For this review, use the dimensioned drawing (mm, ordinates from the lowest corner) and the shaded views. A direction names the side the tool comes from. Coordinates: 2 decimals unless noted, no trailing zeros. Write each loop counter-clockwise with the first axis right and the second up, starting at its lowest first coordinate (ties: lowest second). Pieces come first, ordered by that corner, then holes. Notation, with made-up numbers: (-34.75, 38.5) - (-30.75, 38.5) arc R22 ccw to (-30.75, 44.5) - close; hole circle Ø6 at (-13.5, 65). An arc over 180 degrees is marked (long way). One line per item, written item: value.
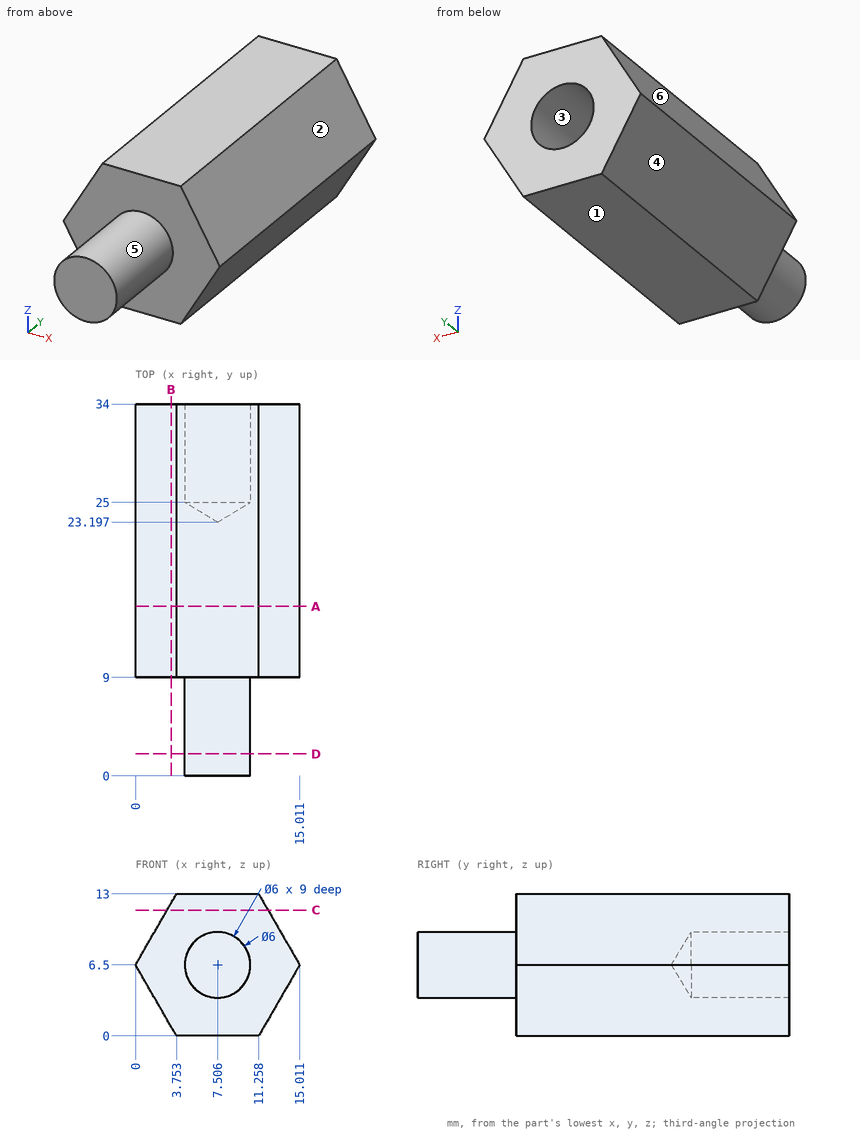
1. Wall thickness on line 1 along Y through (x, z) = (11.75, 12); line 2 along Z through (x, y) = (3.25, 30.5); line 3 along Y through (x, z) = (9.25, 5.75): over which ranges is each line inside the solid? List them lowest first.
Answer block:
line 1: y = 9 to 34
line 2: z = 0.87 to 12.13
line 3: y = 0 to 24.34
2. Mouldability with a two-part tool opening along X and no side actions: class the marked faces 1, 2, 3 and 4 as released by +X, released by -X, zero draft, split by the parting line, or undercut.
Answer block:
face 1: zero draft
face 2: released by +X
face 3: undercut
face 4: released by -X
3. Consider section B-B, the plane x = 3.25. Write out the cut boundary in (y, z).
Answer block:
outline: (9, 0.87) - (34, 0.87) - (34, 12.13) - (9, 12.13) - close
4. Insertion check: pin 1 Ø5 at (x, z) = (3, 1.5) entering from -Y; pin 2 Ø5 at (x, y) = (2.5, 5.5) entering from +Z; pin 3 Ø3 at (y, z) = (3.5, 4.5) entering from -X. Each pin has a flat end and moves straight along its axis. Give the tip position at first contact, or say it passes through.
Answer block:
pin 1: stops at y = 9
pin 2: stops at z = 8.15
pin 3: stops at x = 4.55
5. Consider section D-D, the plane y = 2. Write out the cut boundary in (x, z) (1 decimal).
Answer block:
outline: circle Ø6 at (7.5, 6.5)
6. For the marked faces 5 and 6, list the 3-axis set-ups (+Z, -Z, +X, -X, +Y, -Y) from which the entire face can be reached by the end or side of a thin tool; tool diameter is ignored.
Answer block:
face 5: -Y
face 6: +Z, -X, +Y, -Y
7. Consider section A-A, the plane y = 15.5. Write out the cut boundary in (x, z), then the cut area to 3 significant figures.
Answer block:
outline: (0, 6.5) - (3.75, 0) - (11.26, 0) - (15.01, 6.5) - (11.26, 13) - (3.75, 13) - close
area: 146 mm^2
8. Consider section C-C, the plane z = 11.5. Write out the cut boundary in (x, y) (1 decimal).
Answer block:
outline: (2.9, 9) - (12.1, 9) - (12.1, 34) - (2.9, 34) - close
